Check sheet for the modelled part. Datum: model origin and axes. Units: mm. A direction names the side the tool comes from. Round coordinates to 2 decimals unless told otherwise and drop trailing zeros. Loops run counter-clockwise (first coordinate to the right, second up) from the corner with the lowest first, then second, coordinate; pieces in that order, holes last. Notation, with made-up numbers: (-33.75, 2) - (-6.75, 2) arc R4 cw to (-6.75, 7) - close; hole circle Ø8 at (1, -27). An arc over 180 degrees is marked (long way). Return JSON: item names as keys, results as strings.
from build123d import *

# Parameters (mm, degrees)
CROQUIS1_W              = 90
CROQUIS1_H              = 25
SALIENTE_EXTRUIR1_DEPTH = 0.9
CROQUIS2_R              = 2.15
CORTAR_EXTRUIR1_DEPTH   = 0.9
CROQUIS3_W              = 79.8
CROQUIS3_H              = 9.8
CROQUIS3_R              = 2.15
SALIENTE_EXTRUIR2_DEPTH = 20
CROQUIS4_W              = 79.8
CROQUIS4_H              = 9.8
CROQUIS4_R              = 1.5
SALIENTE_EXTRUIR3_DEPTH = 0.9
CROQUIS5_W              = 5
CROQUIS5_H              = 35
CROQUIS5_R              = 1.5
SALIENTE_EXTRUIR4_DEPTH = 2.7


with BuildPart() as part:
    # Croquis1 → Saliente-Extruir1 (new body)
    with BuildSketch(Plane.XY):
        with Locations((-47.428766378, 9.852941176)):
            Rectangle(CROQUIS1_W, CROQUIS1_H)
    extrude(amount=SALIENTE_EXTRUIR1_DEPTH)

    # Croquis2 → Cortar-Extruir1 (cut)
    with BuildSketch(Plane.XY.offset(0.9)):
        with Locations((-82.428766378, 9.852941176)):
            Circle(CROQUIS2_R)
        with Locations((-72.428766378, 9.852941176)):
            Circle(CROQUIS2_R)
        with Locations((-62.428766378, 9.852941176)):
            Circle(CROQUIS2_R)
        with Locations((-52.428766378, 9.852941176)):
            Circle(CROQUIS2_R)
        with Locations((-42.428766378, 9.852941176)):
            Circle(CROQUIS2_R)
        with Locations((-32.428766378, 9.852941176)):
            Circle(CROQUIS2_R)
        with Locations((-22.428766378, 9.852941176)):
            Circle(CROQUIS2_R)
        with Locations((-12.428766378, 9.852941176)):
            Circle(CROQUIS2_R)
    extrude(amount=-CORTAR_EXTRUIR1_DEPTH, mode=Mode.SUBTRACT)

    # Croquis3 → Saliente-Extruir2 (add)
    with BuildSketch(Plane.XY.offset(0.9)):
        with Locations((-47.428766378, 9.852941176)):
            Rectangle(CROQUIS3_W, CROQUIS3_H)
        with Locations((-12.428766378, 9.852941176)):
            Circle(CROQUIS3_R, mode=Mode.SUBTRACT)
        with Locations((-22.428766378, 9.852941176)):
            Circle(CROQUIS3_R, mode=Mode.SUBTRACT)
        with Locations((-32.428766378, 9.852941176)):
            Circle(CROQUIS3_R, mode=Mode.SUBTRACT)
        with Locations((-42.428766378, 9.852941176)):
            Circle(CROQUIS3_R, mode=Mode.SUBTRACT)
        with Locations((-52.428766378, 9.852941176)):
            Circle(CROQUIS3_R, mode=Mode.SUBTRACT)
        with Locations((-62.428766378, 9.852941176)):
            Circle(CROQUIS3_R, mode=Mode.SUBTRACT)
        with Locations((-72.428766378, 9.852941176)):
            Circle(CROQUIS3_R, mode=Mode.SUBTRACT)
        with Locations((-82.428766378, 9.852941176)):
            Circle(CROQUIS3_R, mode=Mode.SUBTRACT)
    extrude(amount=SALIENTE_EXTRUIR2_DEPTH)

    # Croquis4 → Saliente-Extruir3 (add)
    with BuildSketch(Plane.XY.offset(20.9)):
        with Locations((-47.428766378, 9.852941176)):
            Rectangle(CROQUIS4_W, CROQUIS4_H)
        with Locations((-82.428766378, 9.852941176)):
            Circle(CROQUIS4_R, mode=Mode.SUBTRACT)
        with Locations((-72.428766378, 9.852941176)):
            Circle(CROQUIS4_R, mode=Mode.SUBTRACT)
        with Locations((-62.428766378, 9.852941176)):
            Circle(CROQUIS4_R, mode=Mode.SUBTRACT)
        with Locations((-52.428766378, 9.852941176)):
            Circle(CROQUIS4_R, mode=Mode.SUBTRACT)
        with Locations((-42.428766378, 9.852941176)):
            Circle(CROQUIS4_R, mode=Mode.SUBTRACT)
        with Locations((-32.428766378, 9.852941176)):
            Circle(CROQUIS4_R, mode=Mode.SUBTRACT)
        with Locations((-22.428766378, 9.852941176)):
            Circle(CROQUIS4_R, mode=Mode.SUBTRACT)
        with Locations((-12.428766378, 9.852941176)):
            Circle(CROQUIS4_R, mode=Mode.SUBTRACT)
    extrude(amount=SALIENTE_EXTRUIR3_DEPTH)

    # Croquis5 → Saliente-Extruir4 (add)
    with BuildSketch(Plane.XZ.offset(-4.952941176)):
        with Locations((-82.428766378, 39.3)):
            Rectangle(CROQUIS5_W, CROQUIS5_H)
        with Locations((-82.428766378, 53.8)):
            Circle(CROQUIS5_R, mode=Mode.SUBTRACT)
        with Locations((-72.428766378, 39.3)):
            Rectangle(CROQUIS5_W, CROQUIS5_H)
        with Locations((-72.428766378, 53.8)):
            Circle(CROQUIS5_R, mode=Mode.SUBTRACT)
        with Locations((-62.428766378, 39.3)):
            Rectangle(CROQUIS5_W, CROQUIS5_H)
        with Locations((-62.428766378, 53.8)):
            Circle(CROQUIS5_R, mode=Mode.SUBTRACT)
        with Locations((-52.428766378, 39.3)):
            Rectangle(CROQUIS5_W, CROQUIS5_H)
        with Locations((-52.428766378, 53.8)):
            Circle(CROQUIS5_R, mode=Mode.SUBTRACT)
        with Locations((-42.428766378, 39.3)):
            Rectangle(CROQUIS5_W, CROQUIS5_H)
        with Locations((-42.428766378, 53.8)):
            Circle(CROQUIS5_R, mode=Mode.SUBTRACT)
        with Locations((-32.428766378, 39.3)):
            Rectangle(CROQUIS5_W, CROQUIS5_H)
        with Locations((-32.428766378, 53.8)):
            Circle(CROQUIS5_R, mode=Mode.SUBTRACT)
        with Locations((-22.428766378, 39.3)):
            Rectangle(CROQUIS5_W, CROQUIS5_H)
        with Locations((-22.428766378, 53.8)):
            Circle(CROQUIS5_R, mode=Mode.SUBTRACT)
        with Locations((-12.428766378, 39.3)):
            Rectangle(CROQUIS5_W, CROQUIS5_H)
        with Locations((-12.428766378, 53.8)):
            Circle(CROQUIS5_R, mode=Mode.SUBTRACT)
    extrude(amount=-SALIENTE_EXTRUIR4_DEPTH)


solid = part.part
Q1. Draft check along Y on faces 5 (the face through (-48, 4.953, 16)), 6 (the face through (-23.62, 6.28, 52.89)), 7 (the face through (-20.443, 9.029, 10.304)). Enter one of: released by +Y, released by -Y, zero draft, split by the parting line, or undercut.
Answer key:
{"face 5": "released by -Y", "face 6": "zero draft", "face 7": "undercut"}
Q2. Sectioned sample at B-B (x = -42.5). Enter the section's corners in (y, z).
Answer key:
{"outline": "(-2.65, 0) - (7.7, 0) - (7.7, 20.9) - (8.35, 20.9) - (8.35, 21.8) - (7.65, 21.8) - (7.65, 52.3) - (4.95, 52.3) - (4.95, 0.9) - (-2.65, 0.9) - close; (4.95, 55.3) - (7.65, 55.3) - (7.65, 56.8) - (4.95, 56.8) - close; (11.35, 20.9) - (12, 20.9) - (12, 0) - (22.35, 0) - (22.35, 0.9) - (14.75, 0.9) - (14.75, 21.8) - (11.35, 21.8) - close"}
Q3. Scan lines: probe 1 along Y at (x, z) = (-21.5, 27); probe 2 along Z at (x, y) = (-59, 16); probe 3 along Y at (x, z) = (-84, 12). Record each from-to range of solid material in increasing order. Write a range as [from, to].
Answer key:
{"probe 1": "y = [4.95, 7.65]", "probe 2": "z = [0, 0.9]", "probe 3": "y = [4.95, 8.39], [11.32, 14.75]"}
Q4. Depth check by flat-ended pin: P1, Ø1.5, axis at x = -75.5, z = 32, coming from the +Y side; P2, Ø1.5, axis at x = -76, z = 6, coming from the -Y side; P3, Ø5, axis at x = -12, z = 21, coming from the +Y side. Enter the tip coordinate at first touch or a pass-through.
Answer key:
{"P1": "stops at y = 7.65", "P2": "stops at y = 4.95", "P3": "stops at y = 14.75"}
Q5. Tool access check on faces 1 (the face through (-62, 7.653, 40)), 2 (the face through (-7.529, 10, 11)), 3 (the face through (-14.929, 6, 39)), 4 (the face through (-82.895, 7.754, 10.304)). Record the directions out of +Z, -Z, +X, -X, +Y, -Y that give a thin tool (end or side, any length) a straight path to the whole face; none if there is none.
Answer key:
{"face 1": "+Z, +X, -X, +Y", "face 2": "+Z, +X, +Y, -Y", "face 3": "+Z, +Y, -Y", "face 4": "-Z"}
Q6. Sectioned sample at A-A (z = 38.5). State how many separate pieces and enclosed holes the cut face has, plus the area to 3 significant figures.
Answer key:
{"separate pieces": "8", "enclosed holes": "0", "area": "108 mm²"}
